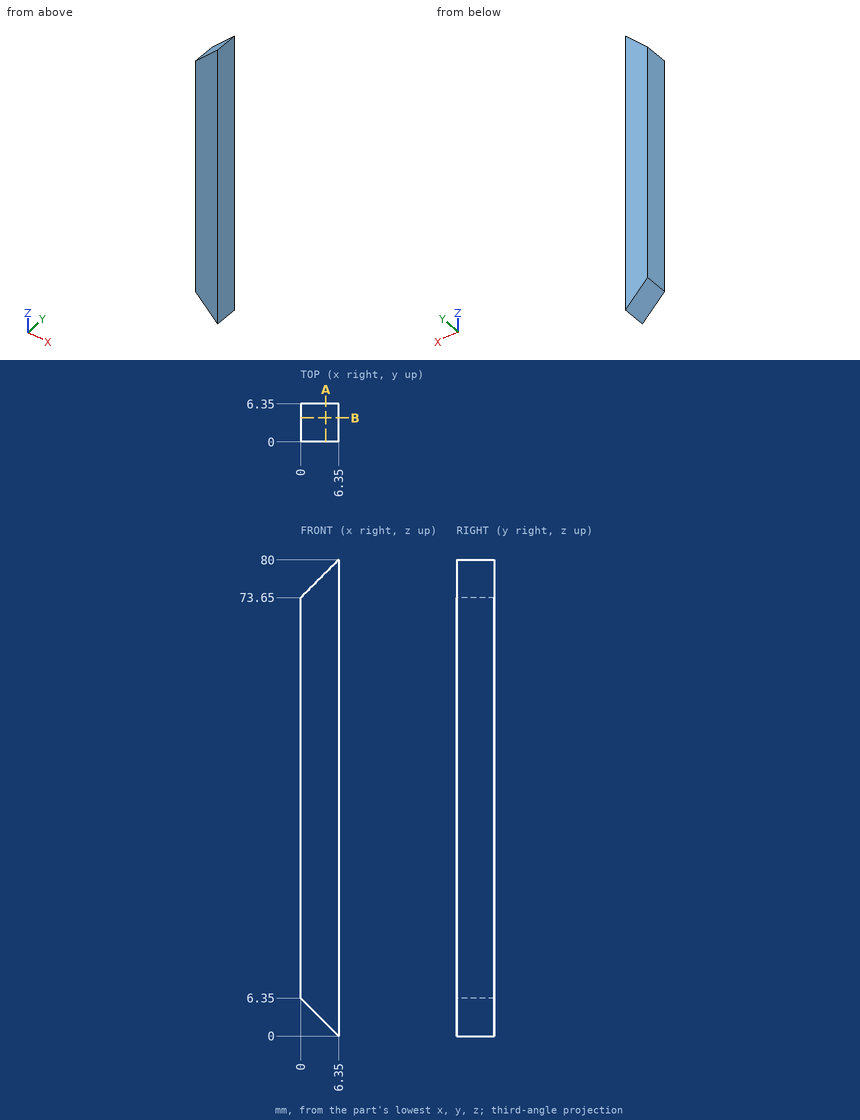
For this review, use the dimensioned drawing (mm, ordinates from the lowest corner) and the shaded views. Round coordinates to 2 decimals unless told otherwise and drop trailing zeros. Write each loop counter-clockwise with the first axis right and the second up, starting at its lowest first coordinate (ties: lowest second). Pieces come first, ordered by that corner, then holes. Notation, with made-up numbers: (56, 6.5) -> (79, 6.5) arc R28 cw to (79, 42.5) -> close; hole circle Ø11 at (73, -12.5). An arc over 180 degrees is marked (long way). One line per item, written item: value. Start each with the question number.
Q1. Add section A-A (x = 4.25). Give the boundary of the cut face in (y, z).
Q2. To check wall thickness, follow probe 1 along Z at (x, y) = (3.5, 1.75); probe 2 along Z at (x, y) = (0.75, 3.5); probe 3 along X at (y, z) = (5.5, 4.5). State the ranges of each line that lie inside material, in increasing order.
Q3. Insertion check: P1, Ø1, axis at x = 5, y = 5, coming from the -Z side. The pin has a flat end and moves straight along its axis. Give the tip position at first contact, or say it passes through.
Q4. Add section B-B (y = 4). Give the boundary of the cut face in (x, z), then the cut area to 3 significant figures.
Response:
1. outline: (0, 2.1) -> (6.35, 2.1) -> (6.35, 77.9) -> (0, 77.9) -> close
2. probe 1: z = 2.85 to 77.15
2. probe 2: z = 5.6 to 74.4
2. probe 3: x = 1.85 to 6.35
3. P1: stops at z = 0.85
4. outline: (0, 6.35) -> (6.35, 0) -> (6.35, 80) -> (0, 73.65) -> close
4. area: 468 mm^2
